Work out the finished part from the listing and answer in its coordinate system (mm). Face numbers are marked on the shaded views. Give positions to 0.01 mm unless a question says otherwise; leave off trailing zeros. Write each loop counter-clockwise with the first axis right and the second up, starting at its lowest first coordinate (ties: lowest second). Pieces come first, ordered by that corner, then holes.
1) Given pin 1 Ø3 at (x, y) = (-24.5, -0.5) entering from +Z; pin 2 Ø1.9 at (x, y) = (-17, 15) entering from +Z, each flat-ended and moving along its own axis, determine where each tip first touches the part or whether it passes through.
2) Find section A-A (z = 7). Count the separate pieces of the cut face and the enclosed holes in it, plus the area to 3 significant figures.
3) Straight lines are drawn through the part: probe 1 along Y at (x, z) = (24.9, 10.75); probe 2 along Y at (x, z) = (-23, 7.25); probe 3 along Z at (x, y) = (-4, 6). For each, find the intervals that lie inside material, in ascending order.
4) Find section D-D (x = 2.5). Determine the outline of the cut face in (y, z).
5) Find section B-B (x = 17). Determine the outline of the cut face in (y, z) (3 decimals).
6) Determine the mould class of the marked faces 1 and 2 for opening direction Z: pulls with the +Z half, pulls with the -Z half, needs draft (parallel to the pull), parting line crosses it, or undercut.
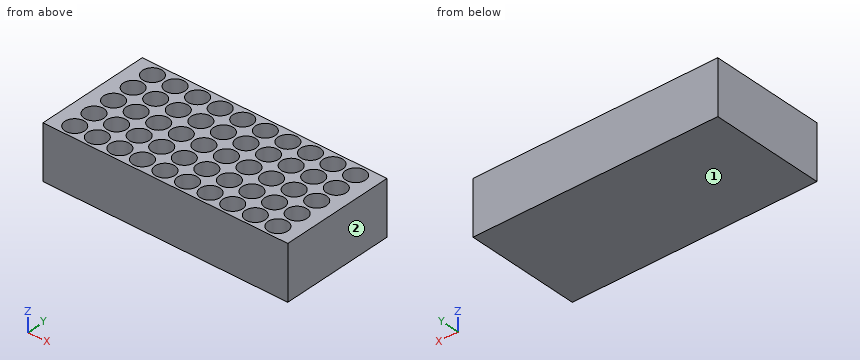
```python
from build123d import *

# Parameters (mm, degrees)
F0_W     = 77
F0_H     = 36
F1_DEPTH = 17
F2_R     = 3.1
F3_DEPTH = 8
F4_R     = 3.1
F5_DEPTH = 11
F6_R     = 3.1
F7_DEPTH = 14


with BuildPart() as f1:
    # F0 (on Top) → F1 (new body)
    with BuildSketch(Plane.XY):
        Rectangle(F0_W, F0_H)
    extrude(amount=F1_DEPTH)

    # F2 (on face) → F3 (cut)
    with BuildSketch(Plane.XY.offset(17)):
        with Locations((-31.9, 14.1)):
            Circle(F2_R)
        with Locations((-24.8, 14.1)):
            Circle(F2_R)
        with Locations((-17.7, 14.1)):
            Circle(F2_R)
        with Locations((-10.6, 14.1)):
            Circle(F2_R)
        with Locations((-3.5, 14.1)):
            Circle(F2_R)
        with Locations((3.6, 14.1)):
            Circle(F2_R)
        with Locations((10.7, 14.1)):
            Circle(F2_R)
        with Locations((17.8, 14.1)):
            Circle(F2_R)
        with Locations((24.9, 14.1)):
            Circle(F2_R)
        with Locations((32, 14.1)):
            Circle(F2_R)
        with Locations((-31.9, -14.1)):
            Circle(F2_R)
        with Locations((-24.8, -14.1)):
            Circle(F2_R)
        with Locations((-17.7, -14.1)):
            Circle(F2_R)
        with Locations((-10.6, -14.1)):
            Circle(F2_R)
        with Locations((-3.5, -14.1)):
            Circle(F2_R)
        with Locations((3.6, -14.1)):
            Circle(F2_R)
        with Locations((10.7, -14.1)):
            Circle(F2_R)
        with Locations((17.8, -14.1)):
            Circle(F2_R)
        with Locations((24.9, -14.1)):
            Circle(F2_R)
        with Locations((32, -14.1)):
            Circle(F2_R)
    extrude(amount=-F3_DEPTH, mode=Mode.SUBTRACT)

    # F4 (on face) → F5 (cut)
    with BuildSketch(Plane.XY.offset(17)):
        with Locations((-31.9, 7.1)):
            Circle(F4_R)
        with Locations((-24.8, 7.1)):
            Circle(F4_R)
        with Locations((-17.7, 7.1)):
            Circle(F4_R)
        with Locations((-10.6, 7.1)):
            Circle(F4_R)
        with Locations((-3.5, 7.1)):
            Circle(F4_R)
        with Locations((3.6, 7.1)):
            Circle(F4_R)
        with Locations((10.7, 7.1)):
            Circle(F4_R)
        with Locations((17.8, 7.1)):
            Circle(F4_R)
        with Locations((24.9, 7.1)):
            Circle(F4_R)
        with Locations((32, 7.1)):
            Circle(F4_R)
        with Locations((-31.9, -7.1)):
            Circle(F4_R)
        with Locations((-24.8, -7.1)):
            Circle(F4_R)
        with Locations((-17.7, -7.1)):
            Circle(F4_R)
        with Locations((-10.6, -7.1)):
            Circle(F4_R)
        with Locations((-3.5, -7.1)):
            Circle(F4_R)
        with Locations((3.6, -7.1)):
            Circle(F4_R)
        with Locations((10.7, -7.1)):
            Circle(F4_R)
        with Locations((17.8, -7.1)):
            Circle(F4_R)
        with Locations((24.9, -7.1)):
            Circle(F4_R)
        with Locations((32, -7.1)):
            Circle(F4_R)
    extrude(amount=-F5_DEPTH, mode=Mode.SUBTRACT)

    # F6 (on face) → F7 (cut)
    with BuildSketch(Plane.XY.offset(17)):
        with Locations((-31.9, 0)):
            Circle(F6_R)
        with Locations((-24.8, 0)):
            Circle(F6_R)
        with Locations((-17.7, 0)):
            Circle(F6_R)
        with Locations((-10.6, 0)):
            Circle(F6_R)
        with Locations((-3.5, 0)):
            Circle(F6_R)
        with Locations((3.6, 0)):
            Circle(F6_R)
        with Locations((10.7, 0)):
            Circle(F6_R)
        with Locations((17.8, 0)):
            Circle(F6_R)
        with Locations((24.9, 0)):
            Circle(F6_R)
        with Locations((32, 0)):
            Circle(F6_R)
    extrude(amount=-F7_DEPTH, mode=Mode.SUBTRACT)


solid = f1.part
```
Results:
1. pin 1: stops at z = 3
1. pin 2: stops at z = 9
2. separate pieces: 1
2. enclosed holes: 30
2. area: 1,870 mm2
3. probe 1: y = -18 to -17.2, -11 to -10.2, -4 to -3.1, 3.1 to 4, 10.2 to 11, 17.2 to 18
3. probe 2: y = -18 to -9.62, -4.58 to -2.52, 2.52 to 4.58, 9.62 to 18
3. probe 3: z = 0 to 6
4. outline: (-18, 0) - (18, 0) - (18, 17) - (17, 17) - (17, 9) - (11.2, 9) - (11.2, 17) - (10, 17) - (10, 6) - (4.2, 6) - (4.2, 17) - (2.9, 17) - (2.9, 3) - (-2.9, 3) - (-2.9, 17) - (-4.2, 17) - (-4.2, 6) - (-10, 6) - (-10, 17) - (-11.2, 17) - (-11.2, 9) - (-17, 9) - (-17, 17) - (-18, 17) - close
5. outline: (-18, 0) - (18, 0) - (18, 17) - (17.095, 17) - (17.095, 9) - (11.105, 9) - (11.105, 17) - (10.095, 17) - (10.095, 6) - (4.105, 6) - (4.105, 17) - (2.995, 17) - (2.995, 3) - (-2.995, 3) - (-2.995, 17) - (-4.105, 17) - (-4.105, 6) - (-10.095, 6) - (-10.095, 17) - (-11.105, 17) - (-11.105, 9) - (-17.095, 9) - (-17.095, 17) - (-18, 17) - close
6. face 1: pulls with the -Z half
6. face 2: needs draft
